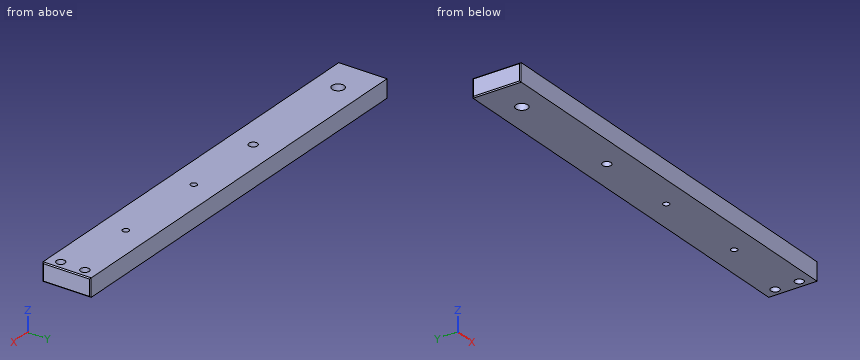
from build123d import *

# Parameters (mm, degrees)
SKETCH1_W                 = 222.25
SKETCH1_H                 = 25.4
BOSS_EXTRUDE1_DEPTH       = 9.525
F_8_CLEARANCE_HOLE1_D     = 4.4958
F_8_CLEARANCE_HOLE1_DEPTH = 25.4
F_8_CLEARANCE_HOLE1_TIP   = 1.350674586
SKETCH5_R                 = 3.1623
CUT_EXTRUDE1_DEPTH        = 9.525
F_8_CLEARANCE_HOLE2_D     = 4.4958
F_8_CLEARANCE_HOLE2_DEPTH = 19.05
F_8_CLEARANCE_HOLE2_TIP   = 1.350674586
CHAMFER1_SIZE             = 0.508
F_4_CLEARANCE_HOLE1_D     = 3.2639


with BuildPart() as part:
    # Sketch1 → Boss-Extrude1 (new body)
    with BuildSketch(Plane.XY):
        with Locations((-111.125, 12.7)):
            Rectangle(SKETCH1_W, SKETCH1_H)
    extrude(amount=BOSS_EXTRUDE1_DEPTH)

    # #8 Clearance Hole1
    with Locations(Plane.XY.offset(9.525)):
        with Locations((-4.7625, 6.35), (-4.7625, 19.05)):
            Hole(F_8_CLEARANCE_HOLE1_D / 2, depth=F_8_CLEARANCE_HOLE1_DEPTH)
            with Locations((0, 0, -(F_8_CLEARANCE_HOLE1_DEPTH + F_8_CLEARANCE_HOLE1_TIP / 2))):  # 118° drill point
                Cone(0, F_8_CLEARANCE_HOLE1_D / 2, F_8_CLEARANCE_HOLE1_TIP, mode=Mode.SUBTRACT)

    # Sketch5 → Cut-Extrude1 (cut)
    with BuildSketch(Plane.XY.offset(9.525)):
        with Locations((-203.2, 12.7)):
            Circle(SKETCH5_R)
    extrude(amount=-CUT_EXTRUDE1_DEPTH, mode=Mode.SUBTRACT)

    # #8 Clearance Hole2
    with Locations(Plane.XY.offset(9.525)):
        with Locations((-139.7, 12.7)):
            Hole(F_8_CLEARANCE_HOLE2_D / 2, depth=F_8_CLEARANCE_HOLE2_DEPTH)
            with Locations((0, 0, -(F_8_CLEARANCE_HOLE2_DEPTH + F_8_CLEARANCE_HOLE2_TIP / 2))):  # 118° drill point
                Cone(0, F_8_CLEARANCE_HOLE2_D / 2, F_8_CLEARANCE_HOLE2_TIP, mode=Mode.SUBTRACT)

    # Chamfer1
    chamfer1_edges = [part.edges().sort_by_distance(p)[0] for p in [
        (-222.25, 12.7, 9.525),
        (0, 12.7, 9.525),
        (-222.25, 12.7, 0),
        (0, 12.7, 0),
        (0, 0, 4.7625),
        (-222.25, 0, 4.7625),
        (-222.25, 25.4, 4.7625),
        (0, 25.4, 4.7625),
    ]]
    chamfer(chamfer1_edges, length=CHAMFER1_SIZE)

    # #4 Clearance Hole1 (through all)
    with Locations(Plane(origin=(0, 0, 0), x_dir=(-1, 0, 0), z_dir=(0, 0, -1))):
        with Locations((95.25, 12.7), (44.45, 12.7)):
            Hole(F_4_CLEARANCE_HOLE1_D / 2)


solid = part.part
Build history of the part. All positions in model axes, mm. Coordinates: 2 decimals unless noted, no trailing zeros. Order: outer loops, then holes, each group sorted by start corner. A loop starts at its lowest first (then second) coordinate and runs counter-clockwise, first axis right, second up. Notation, with made-up numbers: (-6.75, 9.25) - (51.25, 9.25) arc R20 ccw to (51.25, 17.25) - close; hole circle Ø4 at (-5.75, 37.25). An arc over 180 degrees is marked (long way). Write item = value, one per line. Start each with the question number.
1) Saw through at C-C on x = -139.7. Write the cut outline in (y, z) (3 decimals), then the cut area to 3 significant figures.
2) Saw through at B-B on y = 19.05. Write the cut outline in (x, z) (3 decimals).
3) Saw through at A-A on x = -203.2. Write the cut outline in (y, z) (3 decimals).
4) Wall check: line 1 along Y through (x, z) = (-139.7, 3); line 2 along Y through (x, z) = (-44.45, 5); line 3 along X through (y, z) = (6.25, 3). Give the ranges that are in metal, low to high. Write a range as from..to.
From the geometry:
q1.outline = (0, 0) - (10.452, 0) - (10.452, 9.525) - (0, 9.525) - close; (14.948, 0) - (25.4, 0) - (25.4, 9.525) - (14.948, 9.525) - close
q1.area = 199 mm^2
q2.outline = (-222.25, 0.508) - (-221.742, 0) - (-7.01, 0) - (-7.01, 9.525) - (-221.742, 9.525) - (-222.25, 9.017) - close; (-2.515, 0) - (-0.508, 0) - (0, 0.508) - (0, 9.017) - (-0.508, 9.525) - (-2.515, 9.525) - close
q3.outline = (0, 0) - (9.538, 0) - (9.538, 9.525) - (0, 9.525) - close; (15.862, 0) - (25.4, 0) - (25.4, 9.525) - (15.862, 9.525) - close
q4.line_1 = 0..10.45, 14.95..25.4
q4.line_2 = 0..11.07, 14.33..25.4
q4.line_3 = -222.25..-7.01, -2.52..0
